Can you work these out from the model? Positions are in its coordinate system, mm. A direction names the side the tool comes from. Give positions to 0.01 mm unless a question says otherwise; leave off trailing zeros. Loops run counter-clockwise (first coordinate to the right, second up) from the corner with the lowest first, then second, coordinate; pieces in that order, holes last.
from build123d import *

# Parameters (mm, degrees)
SALIENTE_EXTRUIR1_DEPTH = 6
CROQUIS3_W              = 15
CROQUIS3_H              = 15
SALIENTE_EXTRUIR2_DEPTH = 30
CROQUIS4_R              = 5
SALIENTE_EXTRUIR3_DEPTH = 15


with BuildPart() as part:
    # Croquis1 → Saliente-Extruir1 (new body)
    with BuildSketch(Plane(origin=(0, 0, 0), x_dir=(0, 0, -1), z_dir=(1, 0, 0))):
        Polygon((32.5, 0), (-32.5, 0), (-42.5, 100), (42.5, 100), align=None)
    extrude(amount=SALIENTE_EXTRUIR1_DEPTH)

    # Croquis3 → Saliente-Extruir2 (add)
    with BuildSketch(Plane.ZY):
        with Locations((-27.5, 92.5)):
            Rectangle(CROQUIS3_W, CROQUIS3_H)
        with Locations((27.5, 92.5)):
            Rectangle(CROQUIS3_W, CROQUIS3_H)
    extrude(amount=SALIENTE_EXTRUIR2_DEPTH)

    # Croquis4 → Saliente-Extruir3 (add)
    with BuildSketch(Plane(origin=(0, 0, -35), x_dir=(-1, 0, 0), z_dir=(0, 0, -1))):
        with Locations(Location((22.5, 92.538258804, 0), (0, 0, 270))):
            Circle(CROQUIS4_R)
    saliente_extruir3 = extrude(amount=SALIENTE_EXTRUIR3_DEPTH)

    # Simetría1: Saliente-Extruir3 across plane
    add(saliente_extruir3.mirror(Plane.XY))

    # Cortar-Barrer1: sweep along a curve in space
    with BuildLine() as cortar_barrer1_path:
        Line((6, 100, 42.5), (6, 0, 32.5))
    # Croquis7 → Cortar-Barrer1 (sweep, cut)
    with BuildSketch(Plane(origin=(0, 100, 0), x_dir=(1, 0, 0), z_dir=(0, 1, 0))):
        Polygon((0, -42.5), (6, -36.5), (6, -42.5), align=None)
    sweep(path=cortar_barrer1_path.line, mode=Mode.SUBTRACT)

    # Cortar-Barrer2: sweep along a curve in space
    with BuildLine() as cortar_barrer2_path:
        Line((6, 0, -32.5), (6, 100, -42.5))
    # Croquis8 → Cortar-Barrer2 (sweep, cut)
    with BuildSketch(Plane(origin=(0, 100, 0), x_dir=(1, 0, 0), z_dir=(0, 1, 0))):
        Polygon((0, 42.5), (6, 36.5), (6, 42.5), align=None)
    sweep(path=cortar_barrer2_path.line, mode=Mode.SUBTRACT)


solid = part.part
(1) Suppose I cut it at D-D on z = 0.5. List the corners of the cut face in (x, y) for me, plus the area to 3 significant figures.
Returned:
outline: (0, 0) - (6, 0) - (6, 100) - (0, 100) - close
area: 600 mm2
(2) Will these pins go through, and if not, where does the flat tip stop? P1, Ø4.5, axis at x = -21.5, z = -29.5, coming from the -Y side; P2, Ø12, axis at x = -11.5, y = 95, coming from the -Z side; P3, Ø12, axis at y = 35.5, z = 17.5, coming from the -X side.
Returned:
P1: stops at y = 85
P2: stops at z = -35
P3: stops at x = 0
(3) Which directions (+Z, -Z, +X, -X, +Y, -Y) give clear straight access to the entire face, cutting with the end or side of a thin tool? Please do faces 1 (the cylindrical face through (-19.46, 96.51, 42.4)), 2 (the flat face through (-15, 92, 20)), 3 (the flat face through (-15, 85, -28)), 4 (the cylindrical face through (-19.46, 96.51, -42.4)).
Returned:
face 1: +Z
face 2: -X, +Y, -Y
face 3: +Z, -Z, -X, -Y
face 4: -Z
(4) Thinking about a two-plate mould opening in Z: for faces 5 (the flat face through (-15, 85, 27)), 6 (the flat face through (-15, 92, 35)), 7 (the flat face through (-15, 92, -20)), which applies, pulls with the +Z half, pulls with the -Z half, needs draft (parallel to the pull), parting line crosses it, or undercut?
Returned:
face 5: needs draft
face 6: pulls with the +Z half
face 7: undercut
(5) Suppose I cut it at C-C on x = -3.5. List the corners of the cut face in (y, z) for me, plus the area to 3 significant figures.
Returned:
outline: (85, -35) - (100, -35) - (100, -20) - (85, -20) - close; (85, 20) - (100, 20) - (100, 35) - (85, 35) - close
area: 450 mm2
(6) Please list where these lines run through material, in increasing order: probe 1 along Z at (x, y) = (-17.5, 89.5); probe 2 along Y at (x, z) = (-6.5, -25); probe 3 along X at (y, z) = (83, 20).
Returned:
probe 1: z = -35 to -20, 20 to 35
probe 2: y = 85 to 100
probe 3: x = 0 to 6
(7) Suppose I cut it at B-B on y = 30.5. List the corners of the cut face in (x, z) for me, plus the area to 3 significant figures.
Returned:
outline: (0, -35.55) - (6, -29.55) - (6, 29.55) - (0, 35.55) - close
area: 391 mm2
(8) Suppose I cut it at A-A on x = -22.5. List the corners of the cut face in (y, z) for me, plus the area to 3 significant figures.
Returned:
outline: (85, -35) - (87.54, -35) - (87.54, -50) - (97.54, -50) - (97.54, -35) - (100, -35) - (100, -20) - (85, -20) - close; (85, 20) - (100, 20) - (100, 35) - (97.54, 35) - (97.54, 50) - (87.54, 50) - (87.54, 35) - (85, 35) - close
area: 750 mm2
